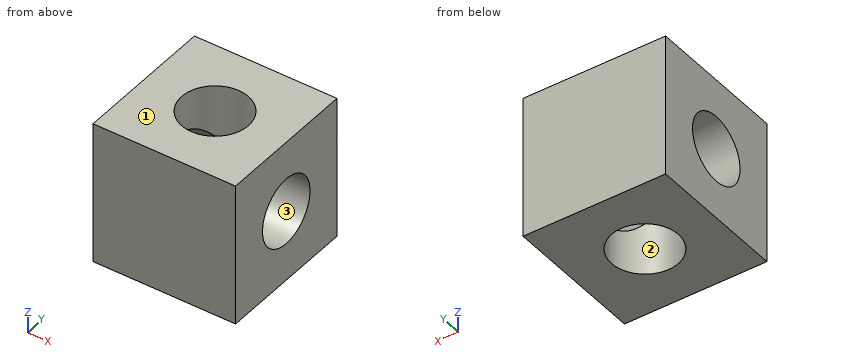
```python
from build123d import *

# Parameters (mm, degrees)
SKETCH1_W           = 20.32
SKETCH1_H           = 20.32
SKETCH1_R           = 4.7625
BOSS_EXTRUDE1_DEPTH = 10.16
SKETCH2_R           = 4.7625
CUT_EXTRUDE1_DEPTH  = 21.32


with BuildPart() as part:
    # Sketch1 → Boss-Extrude1 (new body, symmetric)
    with BuildSketch(Plane.XY):
        Rectangle(SKETCH1_W, SKETCH1_H)
        Circle(SKETCH1_R, mode=Mode.SUBTRACT)
    extrude(amount=BOSS_EXTRUDE1_DEPTH, both=True)

    # Sketch2 → Cut-Extrude1 (cut, through all)
    with BuildSketch(Plane(origin=(10.16, 0, 0), x_dir=(0, 0, -1), z_dir=(1, 0, 0))):
        Circle(SKETCH2_R)
    extrude(amount=-CUT_EXTRUDE1_DEPTH, mode=Mode.SUBTRACT)


solid = part.part
```
Design review of the part built by this model. Coordinates are the model's own, in mm. Face numbers are marked on the shaded views. Give positions to 0.01 mm unless a question says otherwise; leave off trailing zeros. Loops run counter-clockwise (first coordinate to the right, second up) from the corner with the lowest first, then second, coordinate; pieces in that order, holes last. Notation, with made-up numbers: (19.5, -33) -> (43.5, -33) arc R24 cw to (43.5, -4) -> close; hole circle Ø4 at (2, 38). An arc over 180 degrees is marked (long way). Write each question's results on one line, items separated by ' | '.
Q1. Wall thickness on L1, parallel to Y at x = 0, z = 5.75; L2, parallel to Y at x = 7.75, z = 1.5: over which ranges is each line inside the solid? List them lowest first.
Reply:
L1: y = -10.16 to -4.76, 4.76 to 10.16 | L2: y = -10.16 to -4.52, 4.52 to 10.16
Q2. Take a section at B-B, the plane z = -7.75. Write out the cut boundary in (x, y) (1 decimal), plus the area to 3 significant figures.
Reply:
outline: (-10.2, -10.2) -> (10.2, -10.2) -> (10.2, 10.2) -> (-10.2, 10.2) -> close; hole circle Ø9.5 at (0, 0) | area: 342 mm²
Q3. Take a section at A-A, the plane y = 0. Write out the cut boundary in (x, z).
Reply:
outline: (-10.16, -10.16) -> (-4.76, -10.16) -> (-4.76, -4.76) -> (-10.16, -4.76) -> close; (-10.16, 4.76) -> (-4.76, 4.76) -> (-4.76, 10.16) -> (-10.16, 10.16) -> close; (4.76, -10.16) -> (10.16, -10.16) -> (10.16, -4.76) -> (4.76, -4.76) -> close; (4.76, 4.76) -> (10.16, 4.76) -> (10.16, 10.16) -> (4.76, 10.16) -> close
Q4. The part is to be moulded in two halves that separate along Z. For the marked faces 1, 2 and 3, say which applies: +Z half, -Z half, draft (parallel to the pull), parting line (faces both ways), or undercut.
Reply:
face 1: +Z half | face 2: draft | face 3: undercut
